from build123d import *

# Parameters (mm, degrees)
SKETCH1_W                = 25
SKETCH1_H                = 25
BOSS_EXTRUDE1_DEPTH      = 12.5
BOSS_EXTRUDE1_DEPTH_BACK = 12.5
LPATTERN1_COUNT          = 2
LPATTERN1_PITCH          = 15
LPATTERN1_COUNT_DIR2     = 2
LPATTERN1_PITCH_DIR2     = 15
BOSS_EXTRUDE3_START      = 6
SKETCH4_R                = 2.1
BOSS_EXTRUDE3_DEPTH      = 4
BOSS_EXTRUDE5_START      = -6
SKETCH4_5_R              = 2.1
SKETCH4_5_R_2            = 3.5
BOSS_EXTRUDE5_DEPTH      = 6.5


with BuildPart() as part:
    # Sketch1 → Boss-Extrude1 (new, two sides)
    with BuildSketch(Plane.XY) as boss_extrude1_sk:
        Rectangle(SKETCH1_W, SKETCH1_H)
    extrude(amount=BOSS_EXTRUDE1_DEPTH)
    extrude(boss_extrude1_sk.sketch, amount=-BOSS_EXTRUDE1_DEPTH_BACK)

    # Sketch3 → CSK for M3 Oval Head Machine Screw1 (revolve, cut)
    with BuildSketch(Plane(origin=(-7.5, 7.5, 12.5), x_dir=(0, -1, 0), z_dir=(1, 0, 0))):
        Polygon((0, 0), (0, 11.502151548), (2.5, 10), (2.5, 2.860133251), (2.7, 0), align=None)
    csk_for_m3_oval_head_machine_screw1 = revolve(axis=Axis((-7.5, 7.5, 18.85), (0, 0, -1)), mode=Mode.SUBTRACT)

    # LPattern1: CSK for M3 Oval Head Machine Screw1 2 × 2
    with Locations(*[(j * LPATTERN1_PITCH_DIR2, -i * LPATTERN1_PITCH, 0) for i in range(LPATTERN1_COUNT) for j in range(LPATTERN1_COUNT_DIR2) if (i, j) != (0, 0)]):
        add(csk_for_m3_oval_head_machine_screw1, mode=Mode.SUBTRACT)

    # Sketch4 → Boss-Extrude3 (add)
    with BuildSketch(Plane(origin=(0, 0, 0), x_dir=(1, 0, 0), z_dir=(0, 1, 0)).offset(BOSS_EXTRUDE3_START)):
        with BuildLine():
            Line((-22.231166913, -3.489660266), (-12.5, -12.5))
            Line((-12.5, -12.5), (-12.5, 12.5))
            Line((-12.5, 12.5), (-22.231166913, 3.489660266))
            ThreePointArc((-22.231166913, 3.489660266), (-26, 0), (-22.231166913, -3.489660266))
        make_face()
        with Locations(Location((-22.5, 0, 0), (0, 0, 270))):
            Circle(SKETCH4_R, mode=Mode.SUBTRACT)
    extrude(amount=BOSS_EXTRUDE3_DEPTH)

    # Sketch4<5> → Boss-Extrude5 (add)
    with BuildSketch(Plane(origin=(0, 0, 0), x_dir=(1, 0, 0), z_dir=(0, 1, 0)).offset(BOSS_EXTRUDE5_START)):
        with BuildLine():
            ThreePointArc((-22.231166913, 3.489660266), (-24.87792811, 2.568162359), (-26, 0))
            Line((-26, 0), (-22.231166913, 3.489660266))
        make_face()
        with BuildLine():
            Line((-22.231166913, 3.489660266), (-26, 0))
            Line((-26, 0), (-22.231166913, -3.489660266))
            ThreePointArc((-22.231166913, -3.489660266), (-19.931837641, -2.37792811), (-19, 0))
            ThreePointArc((-19, 0), (-19.931837641, 2.37792811), (-22.231166913, 3.489660266))
        make_face()
        with Locations(Location((-22.5, 0, 0), (0, 0, 270))):
            Circle(SKETCH4_5_R, mode=Mode.SUBTRACT)
        with BuildLine():
            Line((-22.231166913, -3.489660266), (-26, 0))
            ThreePointArc((-26, 0), (-24.87792811, -2.568162359), (-22.231166913, -3.489660266))
        make_face()
        with Locations(Location((-22.5, 0, 0), (0, 0, 270))):
            Circle(SKETCH4_5_R)
        with Locations((-22.5, 0)):
            Circle(SKETCH4_5_R_2)
        Polygon((-26, 0), (-12.5, -12.5), (-12.5, 12.5), align=None)
    extrude(amount=-BOSS_EXTRUDE5_DEPTH)

    # Sketch8 → CSK for M3 Oval Head Machine Screw3 (revolve, cut)
    with BuildSketch(Plane(origin=(-22.5, -6, 0), x_dir=(0, 0, 1), z_dir=(1, 0, 0))):
        Polygon((0, 0), (0, 11.502151548), (2.5, 10), (2.5, 2.860133251), (2.7, 0), align=None)
    revolve(axis=Axis((-22.5, 0.35, 0), (0, -1, 0)), mode=Mode.SUBTRACT)


solid = part.part
Can you work these out from the model? Positions are in its coordinate system, mm. A direction names the side the tool comes from. Give positions to 0.01 mm unless a question says otherwise; leave off trailing zeros. Loops run counter-clockwise (first coordinate to the right, second up) from the corner with the lowest first, then second, coordinate; pieces in that order, holes last. Notation, with made-up numbers: (39.25, 67.25) - (69.25, 67.25) arc R17 ccw to (69.25, 89.25) - close; hole circle Ø1 at (15, -29.75). An arc over 180 degrees is marked (long way). One line per item, written item: value.
(1) If we section it at D-D, the plane z = 7: List the corners of the cut face in (x, y) for me.
Verdict:
outline: (-18.44, -12.5) - (12.5, -12.5) - (12.5, 12.5) - (-12.5, 12.5) - (-12.5, 10) - (-18.44, 10) - (-18.44, 6) - (-12.5, 6) - (-12.5, -6) - (-18.44, -6) - close; hole circle Ø5 at (-7.5, -7.5); hole circle Ø5 at (-7.5, 7.5); hole circle Ø5 at (7.5, -7.5); hole circle Ø5 at (7.5, 7.5)
(2) If we mould it in two halves opening along X, with no side actions, what happens to faces 1 (the face through (-7.793, 7.82, 1.259)), 2 (the face through (12.5, 0, 0)), 3 (the face through (-18, 6, 0))? For each: released by +X, released by -X, zero draft, split by the parting line, or undercut.
Verdict:
face 1: undercut
face 2: released by +X
face 3: zero draft
(3) On a 3-axis mill with a long thin cutter (end or side, diameter ignored), from which of +Z, -Z, +X, -X, +Y, -Y can I reach the whole of each face in a straight line? I mean faces 4 (the face through (-25, -11, 0)), 5 (the face through (-25.057, -7.728, -0.336)), 6 (the face through (-17.434, 7.972, 7.932)), 7 (the face through (-5.28, -8.65, 6.12)), 8 (the face through (-16, -6, 0)). Say none if no direction works.
Verdict:
face 4: -Y
face 5: none
face 6: +Z, -X, +Y, -Y
face 7: +Z
face 8: +Z, -Z, -X
(4) If we section it at A-A, the plane z = 4: List the corners of the cut face in (x, y) for me, plus the area to 3 significant figures.
Verdict:
outline: (-21.68, -12.5) - (12.5, -12.5) - (12.5, 12.5) - (-12.5, 12.5) - (-12.5, 10) - (-21.68, 10) - (-21.68, 6) - (-12.5, 6) - (-12.5, -6) - (-21.68, -6) - close; hole circle Ø5 at (-7.5, -7.5); hole circle Ø5 at (-7.5, 7.5); hole circle Ø5 at (7.5, -7.5); hole circle Ø5 at (7.5, 7.5)
area: 643 mm^2
(5) If we section it at C-C, the plane z = -8.25: List the corners of the cut face in (x, y) for me, plus the area to 3 significant figures.
Verdict:
outline: (-17.09, -12.5) - (12.5, -12.5) - (12.5, 12.5) - (-12.5, 12.5) - (-12.5, 10) - (-17.09, 10) - (-17.09, 6) - (-12.5, 6) - (-12.5, -6) - (-17.09, -6) - close
area: 673 mm^2
(6) I'm going to push flat-ended pins straight in: pin 1 (4 mm diameter, centred on x = -16, z = -3, fed in from +Y); pin 2 (6 mm diameter, centred on y = -1.5, z = 5, fed in from -X); pin 3 (4 mm diameter, centred on x = -7.5, y = -7.5, fed in from +Z); pin 4 (6.5 mm diameter, centred on x = 7.5, y = -7.5, fed in from +Z). Where does each tip first touch, or does it pass through?
Verdict:
pin 1: y = 10
pin 2: x = -12.5
pin 3: z = 2.2
pin 4: z = 12.5
(7) I need wall thicknesses on line 1 along Y through (x, z) = (-7.5, 4.5); line 2 along X through (y, z) = (-6.75, 2.75); line 3 along Y through (x, z) = (-16, 2.75). Which ranges of each line are inside material? Lowest first, please.
Verdict:
line 1: -12.5 to -10, -5 to 5, 10 to 12.5
line 2: -24.67 to -9.88, -5.12 to 5.12, 9.88 to 12.5
line 3: -12.5 to -6, 6 to 10
(8) If we section it at B-B, the plane x = -13: List the corners of the cut face in (y, z) for me.
Verdict:
outline: (-12.5, -12.04) - (-6, -12.04) - (-6, 12.04) - (-12.5, 12.04) - close; (6, -12.04) - (10, -12.04) - (10, 12.04) - (6, 12.04) - close
